Geometry check sheet. Reference: drawing and pictorial views, mm from the part's lowest x, y, z. A direction names the side the tool comes from. Give positions to 0.01 mm unless a question says otherwise; leave off trailing zeros. Write each loop counter-clockwise with the first axis right and the second up, starting at its lowest first coordinate (ties: lowest second). Pieces come first, ordered by that corner, then holes. Notation, with made-up numbers: M 7,85.5 L 50,85.5 A14 ccw 50,97.5 Z; hole C 85.5,14.5 d1. An arc over 180 degrees is marked long. One line per item, written item: value. Start each with the question number.
1. Gauge pin test, flat ends, axial feed: pin 1 (8 mm diameter, centred on x = 95, y = 21.5, fed in from -Z); pin 2 (2 mm diameter, centred on x = 96.5, y = 31, fed in from +Z); pin 3 (10 mm diameter, centred on x = 97, z = 83, fed in from -Y) (1 decimal). Record the tip position at first contact, or that the pin passes through.
2. Cross-section at C-C on y = 5.5. Record the cut outline in (x, z).
3. Cross-section at A-A on x = 138. Record the cut outline in (y, z) (1 decimal), then the cut area to 3 significant figures.
4. Scan lines: line 1 (Z direction, x = 137, y = 30); line 2 (Y direction, x = 20.5, z = 163.5) (1 decimal). Record each from-to range of solid material in increasing order.
5. Cross-section at B-B on z = 16. Record the cut outline in (x, y) (1 decimal).
6. Tool access check on the marked faces 1 and 2. Record the directions out of +Z, -Z, +X, -X, +Y, -Y that give a thin tool (end or side, any length) a straight path to the whole face; none if there is none.
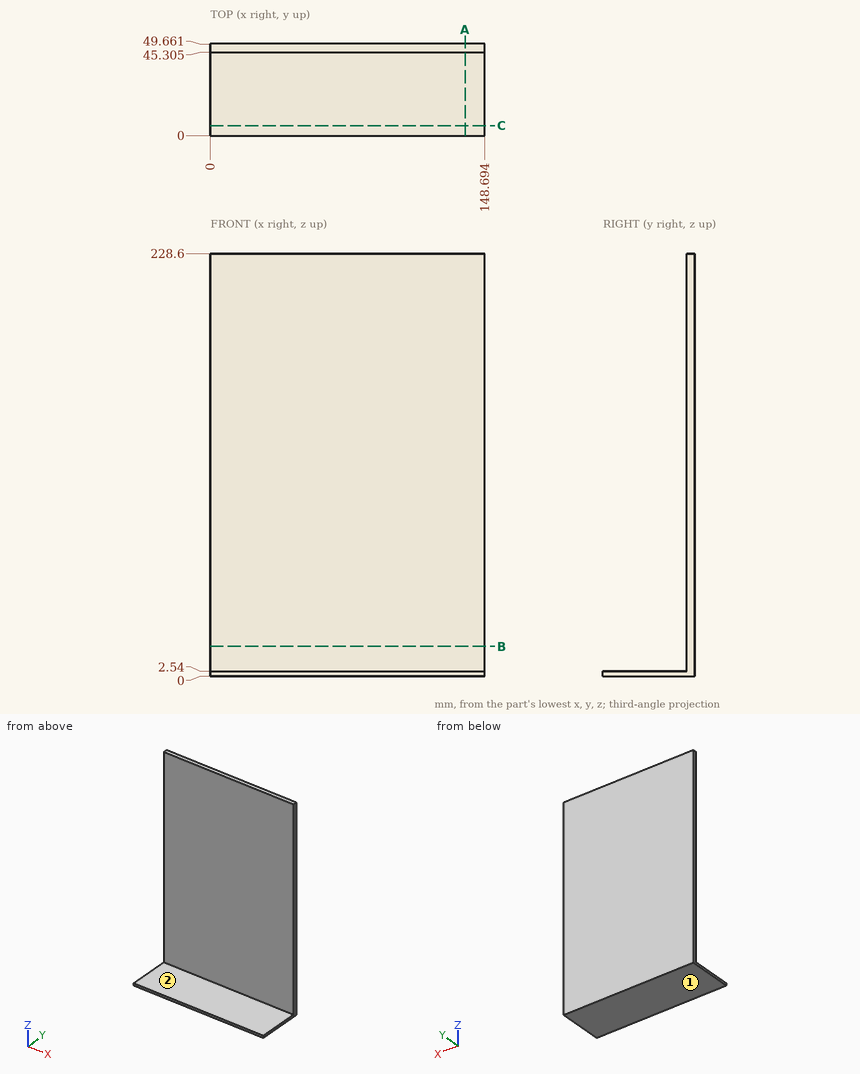
Report:
1. pin 1: stops at z = 0
1. pin 2: stops at z = 2.54
1. pin 3: stops at y = 45.3
2. outline: M 0,0 L 148.69,0 L 148.69,2.54 L 0,2.54 Z
3. outline: M 0,0 L 49.7,0 L 49.7,228.6 L 45.3,228.6 L 45.3,2.5 L 0,2.5 Z
3. area: 1,110 mm^2
4. line 1: z = 0 to 2.54
4. line 2: y = 45.3 to 49.7
5. outline: M 0,45.3 L 148.7,45.3 L 148.7,49.7 L 0,49.7 Z
6. face 1: -Z, +X, -X, +Y, -Y
6. face 2: +Z, +X, -X, -Y
